Autodesk Inventor part; units mm, degrees
ref_plane "YZ Plane" through (0, 0, 0) normal (1, 0, 0) x (0, 1, 0)
ref_plane "XZ Plane" through (0, 0, 0) normal (0, 1, 0) x (-1, 0, 0)
ref_plane "XY Plane" through (0, 0, 0) normal (0, 0, 1) x (1, 0, 0)
sketch "Sketch1" plane through (0, 0, 0) normal (0, 0, 1) x (1, 0, 0)
  line L0 (-50.101, 0.6354) -> (-50.101, 25.1354)
  line L1 (-50.101, 25.1354) -> (-25.801, 25.1354)
  line L2 (-25.801, 25.1354) -> (-25.801, 73.4354)
  line L3 (-25.801, 73.4354) -> (-1.601, 73.4354)
  line L4 (-1.601, 73.4354) -> (-1.601, 25.1354)
  line L5 (-1.601, 25.1354) -> (22.699, 25.1354)
  line L6 (22.699, 25.1354) -> (22.699, 0.6354)
  line L7 (22.699, 0.6354) -> (-50.101, 0.6354)
  line L8 (-23.801, 71.4354) -> (-23.801, 23.1354)
  line L9 (-23.801, 23.1354) -> (-48.101, 23.1354)
  line L10 (-48.101, 23.1354) -> (-48.101, 2.6354)
  line L11 (-48.101, 2.6354) -> (20.699, 2.6354)
  line L12 (20.699, 2.6354) -> (20.699, 23.1354)
  line L13 (20.699, 23.1354) -> (-3.601, 23.1354)
  line L14 (-3.601, 23.1354) -> (-3.601, 71.4354)
  line L15 (-3.601, 71.4354) -> (-23.801, 71.4354)
  line L16 (-13.701, 71.4354) -> (-13.701, 50.8657) construction
  line L17 (-13.701, 2.6354) -> (-13.701, -4.6342) construction
  point P0 (0, 0)
  dimension "d1" = 20.2
  dimension "d2" = 2
  dimension "d3" = 20.5
  dimension "d4" = 68.8
  dimension "d6" = 68.8
extrude "Extrusion1" add sketch "Sketch1" along normal blind 60
sketch "Sketch2" plane through (0, 0, 0) normal (0, 0, -1) x (-1, 0, 0)
  line L0 (1.601, 73.4354) -> (1.601, 25.1354)
  line L1 (25.801, 73.4354) -> (1.601, 73.4354)
  line L2 (25.801, 25.1354) -> (25.801, 73.4354)
  line L3 (50.101, 25.1354) -> (25.801, 25.1354)
  line L4 (50.101, 0.6354) -> (50.101, 25.1354)
  line L5 (-22.699, 0.6354) -> (50.101, 0.6354)
  line L6 (-22.699, 25.1354) -> (-22.699, 0.6354)
  line L7 (1.601, 25.1354) -> (-22.699, 25.1354)
  point P0 (0, 0)
extrude "Extrusion2" add sketch "Sketch2" along normal blind 2
sketch "Sketch3" plane through (0, 0, 0) normal (0, 0, 1) x (1, 0, 0)
  line L0 (-3.601, 71.4354) -> (-7.101, 71.4354)
  line L1 (-7.101, 71.4354) -> (-7.101, 64.9354)
  line L2 (-7.101, 64.9354) -> (-3.601, 64.9354)
  line L3 (-3.601, 64.9354) -> (-3.601, 71.4354)
  line L4 (-48.101, 23.1354) -> (-41.601, 23.1354)
  line L5 (-41.601, 23.1354) -> (-41.601, 19.6354)
  line L6 (-41.601, 19.6354) -> (-48.101, 19.6354)
  line L7 (-48.101, 19.6354) -> (-48.101, 23.1354)
  point P0 (0, 0)
  dimension "d15" = 3.5
  dimension "d16" = 6.5
  dimension "d157" = 6.5
  dimension "d158" = 3.5
extrude "Extrusion3" add sketch "Sketch3" along normal blind 45
sketch "Sketch8" plane through (-25.801, 73.4354, 60) normal (0, 1, 0) x (1, 0, 0)
  line L0 (22.2, 60) -> (22.2, 0)
  line L1 (12.2, -0.1913) -> (22.2, -0.1913)
  line L2 (22.2, -0.1913) -> (22.2, 3.8087)
  line L3 (22.2, 3.8087) -> (12.2, 3.8087)
  line L4 (12.2, 3.8087) -> (12.2, -0.1913)
  point P0 (25.801, 60)
  dimension "d41" = 4
  dimension "d42" = 10
extrude "Extrusion8" cut sketch "Sketch8" against normal blind 2
sketch "Sketch14" plane through (-50.101, 0.6354, 60) normal (0, -1, 0) x (1, 0, 0)
  line L0 (0, 0) -> (-25, 0)
  line L1 (-25, 0) -> (-25, -62)
  line L2 (-25, -62) -> (0, -62)
  line L3 (0, -62) -> (0, 0)
  line L4 (0, -62) -> (0, 0)
  line L5 (0, -31) -> (-8.3028, -31) construction
  line L6 (-25, -31) -> (-20.8134, -31) construction
  circle A0 centre (-15, -5) radius 2.5
  line L7 (72.8, -62) -> (92.8, -62)
  line L8 (92.8, -62) -> (92.8, 0)
  line L9 (92.8, 0) -> (72.8, 0)
  line L10 (72.8, 0) -> (72.8, -62)
  line L11 (72.8, 0) -> (48.5, 0)
  circle A1 centre (82.8, -10) radius 2.5
  circle A2 centre (-15, -57) radius 2.5
  circle A3 centre (82.8, -52) radius 2.5
  point P0 (50.101, -60)
  dimension "d81" = 62
  dimension "d82" = 25
  dimension "d83" = 5
  dimension "d89" = 5
  dimension "d90" = 10
  dimension "d150" = 5
  dimension "d151" = 10
  dimension "d152" = 10
  dimension "d153" = 20
  dimension "d159" = 5
  dimension "d160" = 5
  dimension "d161" = 5
  dimension "d162" = 10
  dimension "d163" = 10
  dimension "d164" = 10
extrude "Extrusion14" add sketch "Sketch14" against normal blind 2
chamfer "Chamfer1" distance 1 angle 45 4 edges at (-67.601, 2.6354, 55) (-67.601, 2.6354, 3) (30.199, 2.6354, 8) (30.199, 2.6354, 50)
sketch "Sketch15" plane through (-50.101, 2.6354, 60) normal (0, 1, 0) x (1, 0, 0)
  line L0 (-6, 47.5876) -> (-22, 47.5876)
  line L1 (-22, 47.5876) -> (-22, 19.5876)
  line L2 (-22, 19.5876) -> (-6, 19.5876)
  line L3 (-6, 19.5876) -> (-6, 47.5876)
  line L4 (0, 0) -> (0, 62)
  point P0 (50.101, 60)
  dimension "d91" = 16
  dimension "d92" = 28
  dimension "d93" = 6
extrude "Extrusion15" add sketch "Sketch15" along normal blind 2
sketch "Sketch16" plane through (-50.101, 0.6354, 60) normal (-1, 0, 0) x (0, 0, 1)
  line L0 (-47.5876, 4) -> (-19.5876, 4)
  line L1 (-59.5876, 15) -> (-29.5876, 15)
  line L2 (-29.5876, 15) -> (-29.5876, 5)
  line L3 (-29.5876, 5) -> (-59.5876, 5)
  line L4 (-59.5876, 5) -> (-59.5876, 15)
  line L5 (-47.5876, 2) -> (-47.5876, 4)
  point P0 (-60, -0.6354)
  dimension "d96" = 18
  dimension "d97" = 30
  dimension "d99" = 1
  dimension "d100" = 10
extrude "Extrusion16" cut sketch "Sketch16" against normal blind 2
sketch "Sketch17" plane through (-50.101, 4.6354, 60) normal (0, 1, 0) x (1, 0, 0)
  circle A0 centre (-19, 44.5876) radius 1.5
  circle A1 centre (-9, 22.5876) radius 1.5
  line L0 (-22, 47.5876) -> (-22, 19.5876)
  line L1 (-6, 47.5876) -> (-22, 47.5876)
  line L2 (-22, 19.5876) -> (-6, 19.5876)
  line L3 (-6, 19.5876) -> (-6, 47.5876)
  point P0 (50.101, 60)
  dimension "d103" = 3
  dimension "d104" = 3
  dimension "d105" = 3
  dimension "d106" = 3
  dimension "d107" = 3
  dimension "d108" = 3
extrude "Extrusion17" cut sketch "Sketch17" against normal blind 4 contours A0 | A1
sketch "Sketch18" plane through (-50.101, 0.6354, 60) normal (0, -1, 0) x (1, 0, 0)
  circle A0 centre (-19, -44.5876) radius 3
  circle A1 centre (-9, -22.5876) radius 3
  circle A2 centre (-19, -44.5876) radius 1.5
  circle A3 centre (-9, -22.5876) radius 1.5
  point P0 (50.101, -60)
  dimension "d111" = 6
  dimension "d112" = 6
extrude "Extrusion18" cut sketch "Sketch18" against normal blind 2
sketch "Sketch19" plane through (-1.601, 25.1354, 60) normal (1, 0, 0) x (0, 0, -1)
  line L0 (10, 32.3) -> (38, 32.3)
  line L1 (38, 32.3) -> (38, 27.3)
  line L2 (38, 27.3) -> (10, 27.3)
  line L3 (10, 27.3) -> (10, 32.3)
  line L4 (0, 48.3) -> (62, 48.3)
  line L5 (0, 0) -> (0, 48.3)
  point P0 (60, -25.1354)
  dimension "d115" = 5
  dimension "d116" = 28
  dimension "d119" = 16
  dimension "d120" = 10
extrude "Extrusion19" add sketch "Sketch19" along normal blind 18
sketch "Sketch20" plane through (-1.601, 57.4354, 50) normal (0, 1, 0) x (1, 0, 0)
  circle A0 centre (15, 25) radius 1.5
  circle A1 centre (5, 3) radius 1.5
  line L0 (0, 28) -> (18, 28)
  line L1 (18, 28) -> (18, 0)
  line L2 (0, 0) -> (18, 0)
  line L3 (0, -10) -> (0, 52)
  point P0 (1.601, 50)
  dimension "d121" = 3
  dimension "d122" = 3
  dimension "d123" = 3
  dimension "d124" = 3
  dimension "d125" = 3
  dimension "d126" = 5
extrude "Extrusion20" cut sketch "Sketch20" against normal blind 10 contours A0 | A1
sketch "Sketch21" plane through (-1.601, 52.4354, 22) normal (0, -1, 0) x (1, 0, 0)
  circle A0 centre (5, 25) radius 2.2
  circle A1 centre (15, 3) radius 2.2
  circle A2 centre (15, 3) radius 1.5
  circle A3 centre (5, 25) radius 1.5
  point P0 (1.601, -22)
  dimension "d129" = 4.4
  dimension "d130" = 4.4
extrude "Extrusion21" cut sketch "Sketch21" against normal blind 2
fillet "Fillet4" radius 2 2 edges at (16.399, 54.9354, 50) (16.399, 54.9354, 22)
sketch "Sketch22" plane through (-1.601, 25.1354, 60) normal (1, 0, 0) x (0, 0, -1)
  line L0 (20, 43.3) -> (60, 43.3)
  line L1 (60, 43.3) -> (60, 33.3)
  line L2 (60, 33.3) -> (20, 33.3)
  line L3 (20, 33.3) -> (20, 43.3)
  line L4 (36, 32.3) -> (12, 32.3)
  line L5 (10, 32.3) -> (10, 27.3)
  point P0 (60, -25.1354)
  dimension "d134" = 1
  dimension "d135" = 10
  dimension "d136" = 40
  dimension "d137" = 10
extrude "Extrusion22" cut sketch "Sketch22" against normal blind 2
sketch "Sketch23" plane through (0, 0, 0) normal (0, 0, 1) x (1, 0, 0)
  line L0 (-48.101, 2.6354) -> (-48.101, 23.1354)
  line L1 (-3.601, 73.4354) -> (-3.601, 23.1354)
  line L2 (-10.601, 22.0354) -> (-3.601, 22.0354)
  line L3 (-3.601, 22.0354) -> (-3.601, 52.0354)
  line L4 (-3.601, 52.0354) -> (-10.601, 52.0354)
  line L5 (-10.601, 52.0354) -> (-10.601, 22.0354)
  line L6 (-28.701, 23.1354) -> (1.299, 23.1354)
  line L7 (1.299, 23.1354) -> (1.299, 16.1354)
  line L8 (1.299, 16.1354) -> (-28.701, 16.1354)
  line L9 (-28.701, 16.1354) -> (-28.701, 23.1354)
  line L10 (-3.601, 23.1354) -> (20.699, 23.1354)
  dimension "d147" = 30
  dimension "d149" = 7
  dimension "d154" = 30
  dimension "d155" = 7
  dimension "d156" = 19.4
extrude "Extrusion23" cut sketch "Sketch23" against normal blind 2
sketch "Sketch24" plane through (-75.101, 0.6354, -2) normal (0, -1, 0) x (1, 0, 0)
  point P0 (75.101, 2)
properties part number "Caja zapato ZOWI DER 2.1"
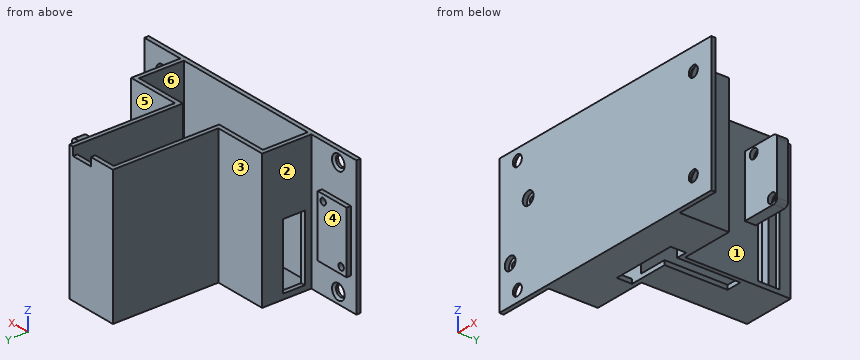
Could you check a few things on this model? Use its own coordinates, in mm. Face numbers are marked on the shaded views. A direction names the side the tool comes from. Round coordinates to 2 decimals unless told otherwise and drop trailing zeros. Order: outer loops, then holes, each group sorted by start corner. A loop starts at its lowest first (then second) coordinate and runs counter-clockwise, first axis right, second up.
Q1. Which directions (+Z, -Z, +X, -X, +Y, -Y) give clear straight access to the entire face, cutting with the end or side of a thin tool? Please do the marked faces 4, 5 and 6.
Geometry says:
face 4: +Z, -Z, -X, +Y
face 5: +Z, -Z, +X
face 6: +Z
Q2. Imagine slicing it at B-B, the plane z = 42. List the corners of the cut face in (x, y) for me, then the cut area to 3 significant figures.
Geometry says:
outline: (-75.1, 0.64) - (42.7, 0.64) - (42.7, 2.64) - (22.7, 2.64) - (22.7, 25.14) - (-1.6, 25.14) - (-1.6, 52.44) - (16.4, 52.44) - (16.4, 57.44) - (-1.6, 57.44) - (-1.6, 73.44) - (-25.8, 73.44) - (-25.8, 25.14) - (-50.1, 25.14) - (-50.1, 2.64) - (-75.1, 2.64) - close; hole (-48.1, 2.64) - (20.7, 2.64) - (20.7, 23.14) - (-3.6, 23.14) - (-3.6, 64.94) - (-7.1, 64.94) - (-7.1, 71.44) - (-23.8, 71.44) - (-23.8, 23.14) - (-41.6, 23.14) - (-41.6, 19.64) - (-48.1, 19.64) - close
area: 792 mm2
Q3. Imagine slicing it at A-A, the plane y = 41.5. List the corners of the cut face in (x, z) for me.
Geometry says:
outline: (-25.8, -2) - (-10.6, -2) - (-10.6, 0) - (-23.8, 0) - (-23.8, 60) - (-25.8, 60) - close; (-3.6, -2) - (-1.6, -2) - (-1.6, 60) - (-3.6, 60) - close
Q4. Imagine slicing it at C-C, the plane x = -21. List the corners of the cut face in (y, z) for me.
Geometry says:
outline: (0.64, -2) - (16.14, -2) - (16.14, 0) - (2.64, 0) - (2.64, 60) - (0.64, 60) - close; (23.14, -2) - (73.44, -2) - (73.44, 60) - (71.44, 60) - (71.44, 0) - (23.14, 0) - close
Q5. Please list where these lines run through material, in increasing order: probe 1 along X at (y, z) = (56.1, 47); probe 2 along Y at (x, z) = (8, 33); probe 3 along Y at (x, z) = (-43.5, 22).
Geometry says:
probe 1: x = -25.8 to -23.8, -3.6 to 1.9, 4.9 to 16.4
probe 2: y = 0.64 to 2.64, 23.14 to 25.14, 52.44 to 57.44
probe 3: y = 0.64 to 2.64, 19.64 to 25.14
Q6. Thinking about a two-plate mould opening in Y: for the marked faces 1, 2 and 3, which applies, released by +Y, released by -Y, zero draft, split by the parting line, or undercut?
Geometry says:
face 1: undercut
face 2: zero draft
face 3: released by +Y
Q7. I'm going to push flat-ended pins straight in: P1, Ø17.5, axis at x = -62, z = 33, coming from the +Y side; P2, Ø22, axis at x = 37, z = 23.5, coming from the +Y side; P3, Ø4, axis at y = 66, z = 17, coming from the +X side. Where does each tip first touch, or does it pass through?
Geometry says:
P1: stops at y = 4.64
P2: stops at y = 2.64
P3: stops at x = -3.6
Q8. Imagine slicing it at D-D, the plane x = -34. List the corners of the cut face in (y, z) for me, then the cut area to 3 significant figures.
Geometry says:
outline: (0.64, -2) - (25.14, -2) - (25.14, 60) - (23.14, 60) - (23.14, 0) - (2.64, 0) - (2.64, 60) - (0.64, 60) - close
area: 289 mm2
